from build123d import *

# Parameters (mm, degrees)
BOSS_EXTRUDE3_DEPTH                          = 10
BOSS_EXTRUDE3_DEPTH_BACK                     = 0.1
SKETCH1_W                                    = 100
SKETCH1_H                                    = 106
SKETCH1_W_2                                  = 76
SKETCH1_H_2                                  = 56
CBORE_FOR_M6_HEX_SOCKET_HEAD_CAP_SCR_2_COUNT = 2
CBORE_FOR_M6_HEX_SOCKET_HEAD_CAP_SCR_2_PITCH = 81
CBORE_FOR_M6_HEX_SOCKET_HEAD_CAP_SCR_3_COUNT = 2
CBORE_FOR_M6_HEX_SOCKET_HEAD_CAP_SCR_3_PITCH = 114.385386776
CBORE_FOR_M6_HEX_SOCKET_HEAD_CAP_SCR_4_COUNT = 2
CBORE_FOR_M6_HEX_SOCKET_HEAD_CAP_SCR_4_PITCH = 80.765194904
SKETCH7_W                                    = 56
SKETCH7_H                                    = 76
BOSS_EXTRUDE4_DEPTH                          = 12
SKETCH8_W                                    = 52
SKETCH8_H                                    = 72
BOSS_EXTRUDE5_DEPTH                          = 1
SKETCH9_W                                    = 52
SKETCH9_H                                    = 72
CUT_EXTRUDE1_DEPTH                           = 1
SKETCH10_W                                   = 52
SKETCH10_H                                   = 62.005454301
CUT_EXTRUDE2_DEPTH                           = 11
SKETCH11_W                                   = 52
SKETCH11_H                                   = 4.999168043
SKETCH11_H_2                                 = 4.995377656
CUT_EXTRUDE3_DEPTH                           = 10
SKETCH12_R                                   = 1.5
CUT_EXTRUDE4_DEPTH                           = 2
SKETCH12_3_R                                 = 1.5
CUT_EXTRUDE5_DEPTH                           = 2
SKETCH14_R                                   = 1.5
CUT_EXTRUDE6_DEPTH                           = 2
SKETCH15_R                                   = 1.5
CUT_EXTRUDE7_DEPTH                           = 2
FILLET2_R                                    = 3


with BuildPart() as part:
    # Sketch1 → Boss-Extrude3 (new, two sides: drawn at the far end of the back side and taken through both)
    # profile 1 of 4: a face of its own
    with BuildSketch(Plane(origin=(0, 0, 0), x_dir=(0, 1, 0), z_dir=(0, 0, 1)).offset(-BOSS_EXTRUDE3_DEPTH_BACK)):
        with Locations((-4.589836902, -8.848323211)):
            Rectangle(SKETCH1_W, SKETCH1_H)
        with Locations((-4.589836902, -8.848323211)):
            Rectangle(SKETCH1_W_2, SKETCH1_H_2, mode=Mode.SUBTRACT)
    # profile 2 of 4: a face of its own
    with BuildSketch(Plane(origin=(0, 0, 0), x_dir=(0, 1, 0), z_dir=(0, 0, 1)).offset(-BOSS_EXTRUDE3_DEPTH_BACK)):
        Polygon((39.410163098, 31.651676789), (39.410163098, -49.348323211), (45.410163098, -61.848323211), (45.410163098, 44.151676789), align=None)
    # profile 3 of 4: a face of its own
    with BuildSketch(Plane(origin=(0, 0, 0), x_dir=(0, 1, 0), z_dir=(0, 0, 1)).offset(-BOSS_EXTRUDE3_DEPTH_BACK)):
        Polygon((33.410163098, 19.151676789), (33.410163098, -36.848323211), (39.410163098, -49.348323211), (39.410163098, 31.651676789), align=None)
    # profile 4 of 4: a face of its own
    with BuildSketch(Plane(origin=(0, 0, 0), x_dir=(0, 1, 0), z_dir=(0, 0, 1)).offset(-BOSS_EXTRUDE3_DEPTH_BACK)):
        Polygon((45.410163098, -61.848323211), (39.410163098, -49.348323211), (39.410163098, -61.848323211), align=None)
    extrude(amount=BOSS_EXTRUDE3_DEPTH + BOSS_EXTRUDE3_DEPTH_BACK)

    # Sketch6 → CBORE for M6 Hex Socket Head Cap Screw2 (revolve, cut)
    with BuildSketch(Plane(origin=(49.348323211, -45.089836902, 10), x_dir=(0, -1, 0), z_dir=(1, 0, 0))):
        Polygon((0, 0), (0, 10.1), (3.3, 10.1), (3.3, 6.4), (5.5, 6.4), (5.5, 0.025), (5.525, 0), align=None)
    cbore_for_m6_hex_socket_head_cap_screw2 = revolve(axis=Axis((49.348323211, -45.089836902, 16.35), (0, 0, -1)), mode=Mode.SUBTRACT)

    # CBORE for M6 Hex Socket Head Cap Scr 2: CBORE for M6 Hex Socket Head Cap Screw2 ×2
    with Locations(*[(0, i * CBORE_FOR_M6_HEX_SOCKET_HEAD_CAP_SCR_2_PITCH, 0) for i in range(1, CBORE_FOR_M6_HEX_SOCKET_HEAD_CAP_SCR_2_COUNT)]):
        add(cbore_for_m6_hex_socket_head_cap_screw2, mode=Mode.SUBTRACT)

    # CBORE for M6 Hex Socket Head Cap Scr 3: CBORE for M6 Hex Socket Head Cap Screw2 ×2
    with Locations(*[Vector(-0.7060796591298035, 0.7081324134391396, 0) * (i * CBORE_FOR_M6_HEX_SOCKET_HEAD_CAP_SCR_3_PITCH) for i in range(1, CBORE_FOR_M6_HEX_SOCKET_HEAD_CAP_SCR_3_COUNT)]):
        add(cbore_for_m6_hex_socket_head_cap_screw2, mode=Mode.SUBTRACT)

    # CBORE for M6 Hex Socket Head Cap Scr 4: CBORE for M6 Hex Socket Head Cap Screw2 ×2
    with Locations(*[(-i * CBORE_FOR_M6_HEX_SOCKET_HEAD_CAP_SCR_4_PITCH, 0, 0) for i in range(1, CBORE_FOR_M6_HEX_SOCKET_HEAD_CAP_SCR_4_COUNT)]):
        add(cbore_for_m6_hex_socket_head_cap_screw2, mode=Mode.SUBTRACT)

    # Sketch7 → Boss-Extrude4 (add)
    with BuildSketch(Plane(origin=(0, 0, -0.1), x_dir=(1, 0, 0), z_dir=(0, 0, -1))):
        with Locations((8.848323211, 4.589836902)):
            Rectangle(SKETCH7_W, SKETCH7_H)
    extrude(amount=-BOSS_EXTRUDE4_DEPTH)

    # Sketch8 → Boss-Extrude5 (add)
    with BuildSketch(Plane.XY.offset(11.9)):
        with Locations((8.848323211, -4.589836902)):
            Rectangle(SKETCH8_W, SKETCH8_H)
    extrude(amount=-BOSS_EXTRUDE5_DEPTH)

    # Sketch9 → Cut-Extrude1 (cut)
    with BuildSketch(Plane.XY.offset(11.9)):
        with Locations((8.848323211, -4.589836902)):
            Rectangle(SKETCH9_W, SKETCH9_H)
    extrude(amount=-CUT_EXTRUDE1_DEPTH, mode=Mode.SUBTRACT)

    # Sketch10 → Cut-Extrude2 (cut)
    with BuildSketch(Plane.XY.offset(10.9)):
        with Locations((8.848323211, -4.587941709)):
            Rectangle(SKETCH10_W, SKETCH10_H)
    extrude(amount=-CUT_EXTRUDE2_DEPTH, mode=Mode.SUBTRACT)

    # Sketch11 → Cut-Extrude3 (cut)
    with BuildSketch(Plane(origin=(0, 0, -0.1), x_dir=(1, 0, 0), z_dir=(0, 0, -1))):
        with Locations((8.848323211, 38.090252881)):
            Rectangle(SKETCH11_W, SKETCH11_H)
        with Locations((8.848323211, -28.91247427)):
            Rectangle(SKETCH11_W, SKETCH11_H_2)
    extrude(amount=-CUT_EXTRUDE3_DEPTH, mode=Mode.SUBTRACT)

    # Sketch12 → Cut-Extrude4 (cut)
    with BuildSketch(Plane.XY.offset(10.9)):
        with Locations((-13.901676789, 28.660163098)):
            Circle(SKETCH12_R)
    extrude(amount=-CUT_EXTRUDE4_DEPTH, mode=Mode.SUBTRACT)

    # Sketch12_3 → Cut-Extrude5 (cut)
    with BuildSketch(Plane.XY.offset(10.9)):
        with Locations((31.598323211, 28.660163098)):
            Circle(SKETCH12_3_R)
    extrude(amount=-CUT_EXTRUDE5_DEPTH, mode=Mode.SUBTRACT)

    # Sketch14 → Cut-Extrude6 (cut)
    with BuildSketch(Plane.XY.offset(10.9)):
        with Locations((-13.901676789, -37.839836902)):
            Circle(SKETCH14_R)
    extrude(amount=-CUT_EXTRUDE6_DEPTH, mode=Mode.SUBTRACT)

    # Sketch15 → Cut-Extrude7 (cut)
    with BuildSketch(Plane.XY.offset(10.9)):
        with Locations((31.598323211, -37.839836902)):
            Circle(SKETCH15_R)
    extrude(amount=-CUT_EXTRUDE7_DEPTH, mode=Mode.SUBTRACT)

    # Fillet2
    fillet2_edges = [part.edges().sort_by_distance(p)[0] for p in [
        (61.848323211, -54.589836902, 4.95),
        (-44.151676789, -54.589836902, 4.95),
        (-44.151676789, 45.410163098, 4.95),
        (61.848323211, 45.410163098, 4.95),
        (-19.151676789, 33.410163098, 10.95),
        (-19.151676789, -42.589836902, 10.95),
        (36.848323211, -42.589836902, 10.95),
        (36.848323211, 33.410163098, 10.95),
    ]]
    fillet(fillet2_edges, radius=FILLET2_R)


solid = part.part
Could you check a few things on this model? Use its own coordinates, in mm. A direction names the side the tool comes from. Give positions to 0.01 mm unless a question says otherwise; leave off trailing zeros. Order: outer loops, then holes, each group sorted by start corner. A loop starts at its lowest first (then second) coordinate and runs counter-clockwise, first axis right, second up. Notation, with made-up numbers: (88.5, 58) - (94.5, 58) arc R20 ccw to (94.5, 77) - close; hole circle Ø2 at (42.5, 84.5). An arc over 180 degrees is marked (long way). One line per item, written item: value. Start each with the question number.
1. Imagine slicing it at D-D on x = 42. List the corners of the cut face in (y, z) for me.
2. For P1, Ø6, axis at x = 49.35, y = -45.09, coming from the -Z side; P2, Ø5.5, axis at x = 47, y = 35, coming from the +Z side; P3, Ø12.5, axis at x = -31.42, y = -45.09, coming from the +Z side; P4, Ø4, axis at x = 5, y = -38.5, coming from the +Z side, each with a flat end and sliding along its axis, tell me the tip position at first contact or that it passes through.
3. If I drill on probe 1 along X at (y, z) = (12, 1.25); probe 2 along Y at (x, z) = (49.5, 1.75); probe 3 along Y at (x, z) = (31, 9.75), over which ranges is the centre line in solid material (lowest first)?
4. Thinking about a two-plate mould opening in X: for faces 1 (the face through (-18.296, -41.688, 10.963)), 2 (the face through (61.848, -5, 5)), 3 (the face through (8, 29, 9.9)), 4 (the face through (10, -54.59, 5)), which applies, +X half, -X half, draft (parallel to the pull), parting line (faces both ways), or undercut?
5. Imagine slicing it at C-C on z = 7.75. List the corners of the cut face in (x, y) for me.
6. For faces 5 (the face through (-26.54, -47.63, 6.83)), 6 (the face through (35.9, 32.6, 11)), 7 (the face through (-18.296, 32.508, 10.963)), which set-ups out of +Z, -Z, +X, -X, +Y, -Y let a thin tool reach every point of the face, with its end or its side?
7. Imagine slicing it at A-A on x = 23.5. List the corners of the cut face in (y, z) for me.
8. Imagine slicing it at B-B on y = 6.5. List the corners of the cut face in (x, z) for me.
Values:
1. outline: (-54.59, -0.1) - (45.41, -0.1) - (45.41, 10) - (-54.59, 10) - close
2. P1: through
2. P2: z = 3.6
2. P3: z = 10
2. P4: z = 10.9
3. probe 1: -44.15 to -17.15, 34.85 to 61.85
3. probe 2: -54.59 to -48.39, -41.79 to 32.61, 39.21 to 45.41
3. probe 3: -54.59 to -40.59, 31.41 to 45.41
4. face 1: -X half
4. face 2: +X half
4. face 3: undercut
4. face 4: draft
5. outline: (-44.15, -51.59) arc R3 ccw to (-41.15, -54.59) - (58.85, -54.59) arc R3 ccw to (61.85, -51.59) - (61.85, 42.41) arc R3 ccw to (58.85, 45.41) - (-41.15, 45.41) arc R3 ccw to (-44.15, 42.41) - close; hole circle Ø11 at (-31.42, -45.09); hole circle Ø11 at (-31.42, 35.91); hole (-17.15, -40.59) - (34.85, -40.59) - (34.85, 31.41) - (-17.15, 31.41) - close; hole circle Ø11 at (49.35, -45.09); hole circle Ø11 at (49.35, 35.91)
6. face 5: +Z
6. face 6: +Z, +X, +Y
6. face 7: +Z, -X, +Y
7. outline: (-54.59, -0.1) - (-40.59, -0.1) - (-40.59, 9.9) - (-35.59, 9.9) - (-35.59, 10.9) - (-40.59, 10.9) - (-40.59, 11.9) - (-42.59, 11.9) - (-42.59, 10) - (-54.59, 10) - close; (26.41, 9.9) - (31.41, 9.9) - (31.41, -0.1) - (45.41, -0.1) - (45.41, 10) - (33.41, 10) - (33.41, 11.9) - (31.41, 11.9) - (31.41, 10.9) - (26.41, 10.9) - close
8. outline: (-44.15, -0.1) - (-17.15, -0.1) - (-17.15, 11.9) - (-19.15, 11.9) - (-19.15, 10) - (-44.15, 10) - close; (34.85, -0.1) - (61.85, -0.1) - (61.85, 10) - (36.85, 10) - (36.85, 11.9) - (34.85, 11.9) - close
